from build123d import *

# Parameters (mm, degrees)
SKETCH_1_W          = 80
SKETCH_1_H          = 60
SKETCH_1_R          = 6.15
EXTRUDE_1_DEPTH     = 5
SKETCH_2_R          = 2.15
CUT_EXTRUDE_1_DEPTH = 68.134361545
SKETCH_3_R          = 2.15
CUT_EXTRUDE_2_DEPTH = 68.134361545
CUT_EXTRUDE_3_DEPTH = 68.134361545
SKETCH_6_R          = 2.15
CUT_EXTRUDE_5_DEPTH = 68.134361545
CUT_EXTRUDE_7_DEPTH = 68.134361545
FILLET_1_R          = 7.5
CUT_EXTRUDE_8_DEPTH = 47.216858546
FILLET_2_R          = 5
FILLET_3_R          = 5


with BuildPart() as part:
    # ｽｹｯﾁ1 → ﾎﾞｽ - 押し出し1 (new body)
    with BuildSketch(Plane.XY):
        with Locations((-19.85, 0)):
            Rectangle(SKETCH_1_W, SKETCH_1_H)
        with Locations((0, 10)):
            Circle(SKETCH_1_R, mode=Mode.SUBTRACT)
    extrude(amount=EXTRUDE_1_DEPTH)

    # ｽｹｯﾁ2 → ｶｯﾄ - 押し出し1 (cut, through all)
    with BuildSketch(Plane.XY.offset(5)):
        with Locations((-54.85, 10)):
            Circle(SKETCH_2_R)
        with Locations(Location((-54.85, -10, 0), (0, 0, 180))):
            Circle(SKETCH_2_R)
        with Locations((-34.85, 10)):
            Circle(SKETCH_2_R)
        with Locations(Location((-34.85, -10, 0), (0, 0, 180))):
            Circle(SKETCH_2_R)
    extrude(amount=-CUT_EXTRUDE_1_DEPTH, mode=Mode.SUBTRACT)

    # ｽｹｯﾁ3 → ｶｯﾄ - 押し出し2 (cut, through all)
    with BuildSketch(Plane.XY.offset(5)):
        with Locations((15.15, 25)):
            Circle(SKETCH_3_R)
        with BuildLine():
            ThreePointArc((15.15, 30), (18.685533906, 28.535533906), (20.15, 25))
            Line((20.15, 25), (20.15, 30))
            Line((20.15, 30), (15.15, 30))
        make_face()
    extrude(amount=-CUT_EXTRUDE_2_DEPTH, mode=Mode.SUBTRACT)

    # ｽｹｯﾁ4 → ｶｯﾄ - 押し出し3 (cut, through all)
    with BuildSketch(Plane.XY.offset(5)):
        Polygon((-59.85, 30), (-59.85, 15), (-29.85, 30), align=None)
        Polygon((-29.85, -30), (-59.85, -15), (-59.85, -30), align=None)
        with BuildLine():
            Line((20.15, 0), (17.493498792, 0))
            ThreePointArc((17.493498792, 0), (15.094907291, -3.347893986), (12.06572435, -6.138178209))
            Line((12.06572435, -6.138178209), (-19.85, -30))
            Line((-19.85, -30), (20.15, -30))
            Line((20.15, -30), (20.15, 0))
        make_face()
        with BuildLine():
            ThreePointArc((20.15, 10), (19.474553919, 4.8265824), (17.493498792, 0))
            Line((17.493498792, 0), (20.15, 0))
            Line((20.15, 0), (20.15, 10))
        make_face()
    extrude(amount=-CUT_EXTRUDE_3_DEPTH, mode=Mode.SUBTRACT)

    # ｽｹｯﾁ6 → ｶｯﾄ - 押し出し5 (cut, through all)
    with BuildSketch(Plane.XY.offset(5)):
        with Locations((-28.669660113, -25)):
            Circle(SKETCH_6_R)
    extrude(amount=-CUT_EXTRUDE_5_DEPTH, mode=Mode.SUBTRACT)

    # ｽｹｯﾁ7 → ｶｯﾄ - 押し出し7 (cut, through all)
    with BuildSketch(Plane.XY.offset(5)):
        with BuildLine():
            Line((-33.038002917, -27.432607888), (-39.85, -15.2))
            Line((-39.85, -15.2), (-29.65, -15.2))
            Line((-29.65, -15.2), (-29.65, 15))
            Line((-29.65, 15), (-10.828193198, 26.993314334))
            ThreePointArc((-10.828193198, 26.993314334), (-6.809164655, 28.964645441), (-2.454078238, 30))
            Line((-2.454078238, 30), (-29.85, 30))
            Line((-29.85, 30), (-59.85, 15))
            Line((-59.85, 15), (-59.85, -15))
            Line((-59.85, -15), (-30.90572732, -29.47213634))
            ThreePointArc((-30.90572732, -29.47213634), (-32.125738379, -28.613242729), (-33.038002917, -27.432607888))
        make_face()
    extrude(amount=-CUT_EXTRUDE_7_DEPTH, mode=Mode.SUBTRACT)

    # ﾌｨﾚｯﾄ1
    # the kernel refuses this fillet: 7.5 mm, written as the material it takes off along each edge
    with BuildSketch(Plane(origin=(-39.85, -15.2, 35.821289963), x_dir=(1, 0, 0), z_dir=(0, 0, -1))) as fillet_1_piece_1:
        with BuildLine():
            CenterArc((12.550603255, 7.122124988), FILLET_1_R, 150.887789783, 100.847129313)
            Line((5.998089047, 10.77103682), (5.867038763, 10.844015057))
            Line((5.867038763, 10.844015057), (-0.131050284, 0.072978237))
            Line((-0.131050284, 0.072978237), (0, -0.15))
            ThreePointArc((0, -0.15), (5.1, -0.15), (10.152987935, -0.1424425))
            Line((10.152987935, -0.1424425), (10.2, 0))
        make_face()
    extrude(amount=66.642579926, mode=Mode.SUBTRACT)
    with BuildSketch(Plane(origin=(-29.65, 15, 15.285449565), x_dir=(0.8433406617465673, 0.5373793150511676, 0), z_dir=(0, 0, -1))) as fillet_1_piece_2:
        with BuildLine():
            CenterArc((FILLET_1_R * 0.548557310151, FILLET_1_R), FILLET_1_R, 212.505415036, 57.494584964)
            Line((-FILLET_1_R * 0.294783351595, FILLET_1_R * 0.462620684949), (-FILLET_1_R * 0.31165016483, FILLET_1_R * 0.451873098648))
            Line((-FILLET_1_R * 0.31165016483, FILLET_1_R * 0.451873098648), (-FILLET_1_R * 0.010971146203, -FILLET_1_R * 0.02))
            Line((-FILLET_1_R * 0.010971146203, -FILLET_1_R * 0.02), (FILLET_1_R * 0.548557310151, -FILLET_1_R * 0.02))
            Line((FILLET_1_R * 0.548557310151, -FILLET_1_R * 0.02), (FILLET_1_R * 0.548557310151, 0))
        make_face()
    extrude(amount=25.570899131, mode=Mode.SUBTRACT)

    # ｽｹｯﾁ8 → ｶｯﾄ - 押し出し8 (cut, through all)
    with BuildSketch(Plane.XY.offset(5)):
        with BuildLine():
            Line((-3.299299523, -7.565945223), (-19.85, -30))
            Line((-19.85, -30), (1.477219454, -14.054684007))
            ThreePointArc((1.477219454, -14.054684007), (0.73895718, -14.088668338), (0, -14.1))
            ThreePointArc((0, -14.1), (-3.659892388, -11.848022648), (-3.299299523, -7.565945223))
        make_face()
        with BuildLine():
            ThreePointArc((0, -5.9), (-1.848022648, -6.340107612), (-3.299299523, -7.565945223))
            ThreePointArc((-3.299299523, -7.565945223), (-3.659892388, -11.848022648), (0, -14.1))
            ThreePointArc((0, -14.1), (0.73895718, -14.088668338), (1.477219454, -14.054684007))
            Line((1.477219454, -14.054684007), (12.06572435, -6.138178209))
            ThreePointArc((12.06572435, -6.138178209), (18.015921371, 0.975085753), (20.15, 10))
            Line((20.15, 10), (20.15, 17.547767201))
            ThreePointArc((20.15, 17.547767201), (16.706289505, 16.278441046), (15.658443273, 12.761006025))
            ThreePointArc((15.658443273, 12.761006025), (12.180106646, -0.220322994), (0, -5.9))
        make_face()
    extrude(amount=-CUT_EXTRUDE_8_DEPTH, mode=Mode.SUBTRACT)

    # ﾌｨﾚｯﾄ2
    fillet_2_edges = [part.edges().sort_by_distance(p)[0] for p in [
        (-19.85, -30, 2.5),
    ]]
    fillet(fillet_2_edges, radius=FILLET_2_R)

    # ﾌｨﾚｯﾄ3
    fillet_3_edges = [part.edges().sort_by_distance(p)[0] for p in [
        (20.15, 17.547767201, 2.5),
    ]]
    fillet(fillet_3_edges, radius=FILLET_3_R)


solid = part.part
The listing builds one solid part. Answer for the finished solid, in the listing's coordinates (mm). A direction names the side the tool comes from. Round coordinates to 2 decimals unless told otherwise and drop trailing zeros. Write each loop counter-clockwise with the first axis right and the second up, starting at its lowest first coordinate (ties: lowest second). Pieces come first, ordered by that corner, then holes. Notation, with made-up numbers: M 41.25,23 L 99.25,23 A11 cw 99.25,37 Z; hole C 64.25,-35 d9. An arc over 180 degrees is marked long. Write each question's results on one line, items separated by ' | '. Start each with the question number.
Item 1: The mould has two halves that part along Y. Classify faces 1 (the cylindrical face through (15.996, 15.238, 2.535)), 2 (the cylindrical face through (-28.75, 14.45, 2.54)), 3 (the flat face through (-26, -30, 2)): +Y half, -Y half, draft (parallel to the pull), parting line (faces both ways), or undercut.
Item 2: Find section A-A on y = 10. Write down the section's boundary in (x, z), and give its area (3 significant figures).
Item 3: Straight lines are drawn through the part: probe 1 along X at (y, z) = (11.5, 2.9); probe 2 along Y at (x, z) = (-28, 3.4); probe 3 along Y at (x, z) = (-9, 2.7). For each, find the intervals that lie inside material, in ascending order.
Item 4: Find section C-C on y = -25. Write down the section's boundary in (x, z).
Item 5: Find section B-B on z = 2.6. Write down the section's boundary in (x, y).
Item 6: Find section D-D on x = -12. Write down the section's boundary in (y, z), and give its area (3 significant figures).
Item 7: Which of the six approach directions +Z, -Z, +X, -X, +Y, -Y give full straight-line access (tool end or side, diameter ignored) to faces 4 (the flat face through (-29.65, -2, 3)), 5 (the flat face through (-33.44, -26.71, 2.54))?
Item 8: Given pin 1 Ø7.5 at (x, y) = (0, 10) entering from -Z; pin 2 Ø1 at (x, z) = (-6.5, 4.5) entering from -Y; pin 3 Ø1.5 at (y, z) = (-6, 3) entering from -X; pin 4 Ø1.5 at (x, z) = (-22.5, 1.5) entering from +Y, each flat-ended and moving along its own axis, determine where each tip first touches the part or whether it passes through.
Answer block:
1) face 1: undercut | face 2: +Y half | face 3: -Y half
2) outline: M -29.65,0 L -6.15,0 L -6.15,5 L -29.65,5 Z; M 6.15,0 L 15.9,0 L 15.9,5 L 6.15,5 Z | area: 166 mm²
3) probe 1: x = -29.62 to -5.96, 5.96 to 15.83 | probe 2: y = -30 to -27.04, -22.96 to 15.58 | probe 3: y = -15.29 to 28.03
4) outline: M -34.31,0 L -30.82,0 L -30.82,5 L -34.31,5 Z; M -26.52,0 L -16.16,0 L -16.16,5 L -26.52,5 Z
5) outline: M -33.85,-25.97 L -33.04,-27.43 A5 ccw -30.91,-29.47 L -29.85,-30 L -22.37,-30 A5 ccw -18.35,-27.97 L -3.3,-7.57 A4.1 cw 0,-5.9 A15.9 ccw 15.66,12.76 A4.1 cw 17.65,17.02 A5 ccw 20.15,21.36 L 20.15,25 A5 ccw 15.15,30 L -2.45,30 A20.15 ccw -10.83,26.99 L -26.18,17.21 A7.5 ccw -29.65,10.89 L -29.65,-15.2 A7.5 ccw Z; hole C -28.67,-25 d4.3; hole C 0,10 d12.3; hole C 15.15,25 d4.3
6) outline: M -19.36,0 L 26.25,0 L 26.25,5 L -19.36,5 Z | area: 228 mm²
7) face 4: +Z, -Z, -X, +Y | face 5: +Z, -Z, -X, -Y
8) pin 1: passes through | pin 2: stops at y = -12.58 | pin 3: stops at x = -29.65 | pin 4: stops at y = 20.03
